The listing builds one solid part. Answer for the finished solid, in the listing's coordinates (mm). Give positions to 0.01 mm unless a question says otherwise; leave off trailing zeros. Loops run counter-clockwise (first coordinate to the right, second up) from the corner with the lowest first, then second, coordinate; pieces in that order, holes last. Notation, with made-up numbers: (60, 59.5) - (96, 59.5) arc R27 ccw to (96, 91.5) - close; hole circle Ø8 at (-22, 29.5). An arc over 180 degrees is marked (long way). Write each question's results on one line, items separated by ' | '.
from build123d import *

# Parameters (mm, degrees)
F2_R = 0.99999
F3_R = 5


# Not quite as in the source:
# - a fillet or chamfer is up to 0.001 mm smaller than in the source, because OpenCascade refuses the exact size


with BuildPart() as f1:
    # F0 (on Front) → F1 (revolve)
    with BuildSketch(Plane.XZ):
        Polygon((0, 4.25), (0, 2.25), (14.4355785643, 2.25), (37.4355785643, 2.25), (37.4355785643, 8.3307377657), (14.4355785643, 9.5361166892), (10, 4.25), align=None)
    revolve(axis=Axis((-40, 0, 0), (1, 0, 0)))

    # F2 (radius 1 in the source; OpenCascade refuses exactly that, so slightly less here)
    f2_edges = [f1.edges().sort_by_distance(p)[0] for p in [
        (0, 0, -4.25),
        (37.435579, 0, -8.330738),
        (37.435579, 0, -2.25),
        (0, 0, -2.25),
    ]]
    fillet(f2_edges, radius=F2_R)

    # F3
    f3_edges = [f1.edges().sort_by_distance(p)[0] for p in [
        (14.435579, 0, -9.536117),
        (10, 0, -4.25),
    ]]
    fillet(f3_edges, radius=F3_R)


solid = f1.part
Item 1: Find the intervals of material crossed by line 1 along Y through (x, z) = (26, 0); line 2 along Z through (x, y) = (22.5, -1.75); line 3 along Z through (x, y) = (23, 0), in increasing order. Write a range as [from, to].
Values found:
line 1: y = [-8.93, -2.25], [2.25, 8.93] | line 2: z = [-8.94, -1.41], [1.41, 8.94] | line 3: z = [-9.09, -2.25], [2.25, 9.09]
Item 2: A cutting plane is placed at A-A, the plane x = 3.5. Determine the outline of the cut face in (y, z), plus the area to 3 significant figures.
Values found:
outline: circle Ø8.5 at (0, 0); hole circle Ø4.5 at (0, 0) | area: 40.8 mm²
Item 3: For a pull along Z with two mould halves and no side action, classify faces 1 (the face through (37.436, 3, -2)), 2 (the face through (18.97, -2.23, -0.29)), 3 (the face through (4.288, -1.277, 4.054)) as released by +Z, released by -Z, zero draft, split by the parting line, or undercut.
Values found:
face 1: zero draft | face 2: undercut | face 3: split by the parting line
Item 4: A cutting plane is placed at B-B, the plane x = 34. Determine the outline of the cut face in (y, z), plus the area to 3 significant figures.
Values found:
outline: circle Ø17.02 at (0, 0); hole circle Ø4.5 at (0, 0) | area: 212 mm²
Item 5: Flat-ended cylindrical pins translate along their axes: P1, Ø1.5, axis at x = 17, z = -5, coming from the +Y side; P2, Ø4, axis at x = 18, z = 4.5, coming from the -Y side; P3, Ø1.5, axis at y = -1, z = 4, coming from the -X side. Find the tip coordinate at first contact, or state that the pin passes through.
Values found:
P1: stops at y = 8.39 | P2: stops at y = -9.02 | P3: stops at x = 0.01
